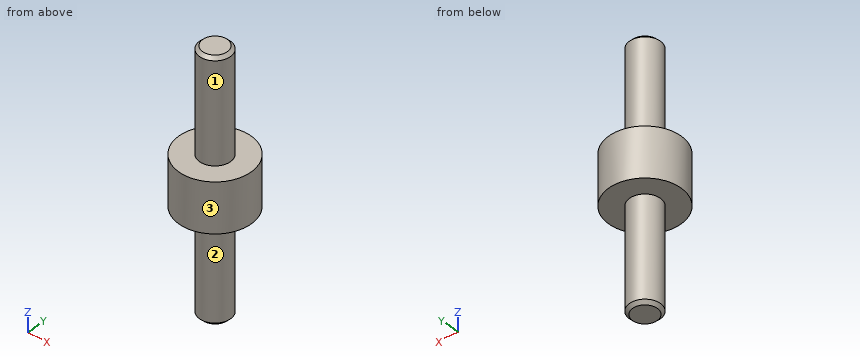
Autodesk Inventor part; units mm, degrees
ref_plane "YZ Plane" through (0, 0, 0) normal (1, 0, 0) x (0, 1, 0)
ref_plane "XZ Plane" through (0, 0, 0) normal (0, 1, 0) x (-1, 0, 0)
ref_plane "XY Plane" through (0, 0, 0) normal (0, 0, 1) x (1, 0, 0)
sketch "Boceto1" plane through (0, 0, 0) normal (0, 1, 0) x (-1, 0, 0)
  line L0 (0, 12.4) -> (1.5, 12.4)
  line L1 (1.5, 12.4) -> (1.5, 2.4)
  line L2 (1.5, 2.4) -> (3.5, 2.4)
  line L3 (3.5, 2.4) -> (3.5, -2.4)
  line L4 (3.5, -2.4) -> (1.5, -2.4)
  line L5 (1.5, -2.4) -> (1.5, -12.4)
  line L6 (1.5, -12.4) -> (0, -12.4)
  line L7 (0, -12.4) -> (0, 12.4)
  point P0 (0, 0)
  point P1 (0, 0)
  dimension "d0" = 7
  dimension "d1" = 3
  dimension "Dedos" = 4.8
  dimension "R" = 10
revolve "Revolución1" add sketch "Boceto1" angle 360 about axis through (0, 0, -12.4) along (0, 0, 1)
thread "Rosca2"
thread "Rosca3"
chamfer "Chaflán1" distance 0.3067 angle 45 2 edges at (1.5, 0, 12.4) (1.5, 0, -12.4)
properties part number "Clavija" material "Aluminum 7075"
Geometry check sheet. Reference: the model listing, model coordinates, mm. Face numbers are marked on the shaded views. A direction names the side the tool comes from. Give positions to 0.01 mm unless a question says otherwise; leave off trailing zeros. Loops run counter-clockwise (first coordinate to the right, second up) from the corner with the lowest first, then second, coordinate; pieces in that order, holes last. Notation, with made-up numbers: (73.5, -1) -> (129.5, -1) arc R21 cw to (129.5, 12) -> close; hole circle Ø11 at (34.25, 30). An arc over 180 degrees is marked (long way). Answer in a Markdown table with one row per item. Add a question column.
1) Gauge pin test, flat ends, axial feed: P1, Ø4, axis at x = 0, y = -1.5, coming from the -Z side; P2, Ø1, axis at x = 1, z = -8, coming from the +Y side. Record the tip position at first contact, or that the pin passes through.
2) Material ranges on probe 1 along Y at (x, z) = (0, 10); probe 2 along Z at (x, y) = (2.5, -1), recorded low to high. Write a range as from..to.
3) Cross-section at D-D on y = -2.25. Record the boundary of the cut face in (x, z).
4) Cross-section at A-A on x = 0. Record the boundary of the cut face in (y, z).
5) Cross-section at C-C on z = 9.25. Record the boundary of the cut face in (x, y), and give its area (3 significant figures).
6) Set-up check for the marked faces 1, 2 and 3: record each of +Z, -Z, +X, -X, +Y, -Y from which the full face is reachable in a straight line by a thin tool's end or side.
Outcome:
| question | item | result |
|---|---|---|
| 1 | P1 | stops at z = -12.4 |
| 1 | P2 | stops at y = 1.41 |
| 2 | probe 1 | y = -1.5..1.5 |
| 2 | probe 2 | z = -2.4..2.4 |
| 3 | outline | (-2.68, -2.4) -> (2.68, -2.4) -> (2.68, 2.4) -> (-2.68, 2.4) -> close |
| 4 | outline | (-3.5, -2.4) -> (-1.5, -2.4) -> (-1.5, -12.09) -> (-1.19, -12.4) -> (1.19, -12.4) -> (1.5, -12.09) -> (1.5, -2.4) -> (3.5, -2.4) -> (3.5, 2.4) -> (1.5, 2.4) -> (1.5, 12.09) -> (1.19, 12.4) -> (-1.19, 12.4) -> (-1.5, 12.09) -> (-1.5, 2.4) -> (-3.5, 2.4) -> close |
| 5 | outline | circle Ø3 at (0, 0) |
| 5 | area | 7.07 mm^2 |
| 6 | face 1 | +Z |
| 6 | face 2 | -Z |
| 6 | face 3 | +Z, -Z |
